Could you check a few things on this model? Use its own coordinates, in mm. A direction names the side the tool comes from. Round coordinates to 2 decimals unless told otherwise and drop trailing zeros. Write each loop counter-clockwise with the first axis right and the second up, starting at its lowest first coordinate (ties: lowest second). Pieces come first, ordered by that corner, then holes. Notation, with made-up numbers: (-26.75, 11) -> (23.25, 11) arc R16 ccw to (23.25, 19) -> close; hole circle Ø11 at (79, -10.5). An arc over 180 degrees is marked (long way). Answer in a Markdown table with one row per item.
from build123d import *

# Parameters (mm, degrees)
F0_W     = 85.6
F0_H     = 17
F1_DEPTH = 1.5875
F2_R     = 2


# Not quite as in the source:
# - a length typed as a fraction of an inch, garbled in the dataset ("3 / 203.2 mm" for 3/8 in), is restored


with BuildPart() as f1:
    # F0 (on Top) → F1 (new body)
    with BuildSketch(Plane.XY):
        Rectangle(F0_W, F0_H)
        with BuildLine():
            ThreePointArc((-35.3, -5.5), (-36.8, -7), (-38.3, -5.5))
            Line((-38.3, -5.5), (-38.3, -3.5))
            ThreePointArc((-38.3, -3.5), (-36.8, -2), (-35.3, -3.5))
            Line((-35.3, -3.5), (-35.3, -5.5))
        make_face(mode=Mode.SUBTRACT)
        with BuildLine():
            ThreePointArc((35.3, -3.5), (36.8, -2), (38.3, -3.5))
            Line((38.3, -3.5), (38.3, -5.5))
            ThreePointArc((38.3, -5.5), (36.8, -7), (35.3, -5.5))
            Line((35.3, -5.5), (35.3, -3.5))
        make_face(mode=Mode.SUBTRACT)
        with BuildLine():
            ThreePointArc((-38.3, 5.5), (-36.8, 7), (-35.3, 5.5))
            Line((-35.3, 5.5), (-35.3, 3.5))
            ThreePointArc((-35.3, 3.5), (-36.8, 2), (-38.3, 3.5))
            Line((-38.3, 3.5), (-38.3, 5.5))
        make_face(mode=Mode.SUBTRACT)
        with BuildLine():
            Line((35.3, 3.5), (35.3, 5.5))
            ThreePointArc((35.3, 5.5), (36.8, 7), (38.3, 5.5))
            Line((38.3, 5.5), (38.3, 3.5))
            ThreePointArc((38.3, 3.5), (36.8, 2), (35.3, 3.5))
        make_face(mode=Mode.SUBTRACT)
    extrude(amount=F1_DEPTH)

    # F2
    f2_edges = [f1.edges().sort_by_distance(p)[0] for p in [
        (-42.8, -8.5, 0.79375),
        (-42.8, 8.5, 0.79375),
        (42.8, 8.5, 0.79375),
        (42.8, -8.5, 0.79375),
    ]]
    fillet(f2_edges, radius=F2_R)


solid = f1.part
1) Thinking about a two-plate mould opening in Y: for faces 1 (the face through (36.8, -2, 0.8)), 2 (the face through (-42.8, 0, 1)), 3 (the face through (-35.3, 5, 1)), 4 (the face through (-1, 8.5, 1)), which applies, +Y half, -Y half, draft (parallel to the pull), parting line (faces both ways), or undercut?
Findings:
| item | result |
|---|---|
| face 1 | undercut |
| face 2 | draft |
| face 3 | undercut |
| face 4 | +Y half |
2) For faces 5 (the face through (38.3, -4, 1)), 6 (the face through (-1, -8.5, 1)), which set-ups out of +Z, -Z, +X, -X, +Y, -Y let a thin tool reach every point of the face, with its end or its side?
Findings:
| item | result |
|---|---|
| face 5 | +Z, -Z |
| face 6 | +Z, -Z, +X, -X, -Y |
3) Please list where these lines run through material, in increasing order: line 1 (Y direction, x = 37, z = 0.3); line 2 (X direction, y = -3.75, z = 1.3); line 3 (X direction, y = 6.25, z = 0.45).
Findings:
| item | result |
|---|---|
| line 1 | y = -8.5 to -6.99, -2.01 to 2.01, 6.99 to 8.5 |
| line 2 | x = -42.8 to -38.3, -35.3 to 35.3, 38.3 to 42.8 |
| line 3 | x = -42.8 to -38.1, -35.5 to 35.5, 38.1 to 42.8 |
4) Imagine slicing it at A-A, the plane y = 4.5. Please give me the cut outline in (x, z).
Findings:
| item | result |
|---|---|
| outline | (-42.8, 0) -> (-38.3, 0) -> (-38.3, 1.59) -> (-42.8, 1.59) -> close; (-35.3, 0) -> (35.3, 0) -> (35.3, 1.59) -> (-35.3, 1.59) -> close; (38.3, 0) -> (42.8, 0) -> (42.8, 1.59) -> (38.3, 1.59) -> close |
5) Imagine slicing it at B-B, the plane z = 1.15. Please give me the cut outline in (x, y), plus the area to 3 significant figures.
Findings:
| item | result |
|---|---|
| outline | (-42.8, -6.5) arc R2 ccw to (-40.8, -8.5) -> (40.8, -8.5) arc R2 ccw to (42.8, -6.5) -> (42.8, 6.5) arc R2 ccw to (40.8, 8.5) -> (-40.8, 8.5) arc R2 ccw to (-42.8, 6.5) -> close; hole (-38.3, -5.5) arc R1.5 ccw to (-35.3, -5.5) -> (-35.3, -3.5) arc R1.5 ccw to (-38.3, -3.5) -> close; hole (-38.3, 3.5) arc R1.5 ccw to (-35.3, 3.5) -> (-35.3, 5.5) arc R1.5 ccw to (-38.3, 5.5) -> close; hole (35.3, -5.5) arc R1.5 ccw to (38.3, -5.5) -> (38.3, -3.5) arc R1.5 ccw to (35.3, -3.5) -> close; hole (35.3, 3.5) arc R1.5 ccw to (38.3, 3.5) -> (38.3, 5.5) arc R1.5 ccw to (35.3, 5.5) -> close |
| area | 1,400 mm^2 |
6) Imagine slicing it at C-C, the plane x = -36.8. Please give me the cut outline in (y, z).
Findings:
| item | result |
|---|---|
| outline | (-8.5, 0) -> (-7, 0) -> (-7, 1.59) -> (-8.5, 1.59) -> close; (-2, 0) -> (2, 0) -> (2, 1.59) -> (-2, 1.59) -> close; (7, 0) -> (8.5, 0) -> (8.5, 1.59) -> (7, 1.59) -> close |
